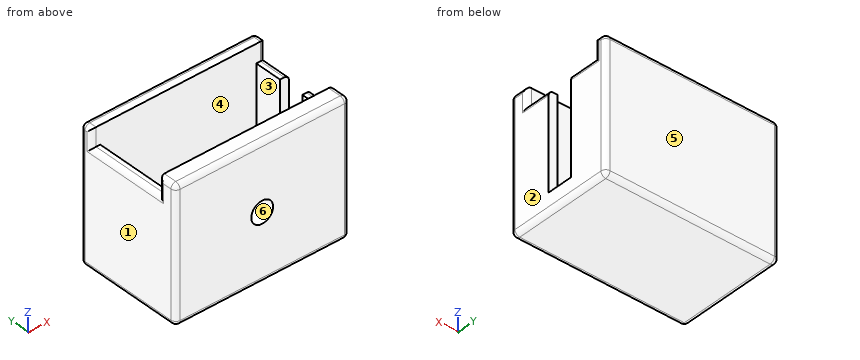
```python
from build123d import *

# Parameters (mm, degrees)
F0_W     = 46.0375
F0_H     = 28.575
F1_DEPTH = 4.7625
F3_DEPTH = 30.2895
F2_W     = 2.38125
F2_H     = 20.6375
F4_DEPTH = 25.4
F6_DEPTH = 2.38125
F8_D     = 5.7658
F8_DEPTH = 4.7625
F8_TIP   = 1.7322210786
F9_R     = 1.27


# Not quite as in the source:
# - a feature names something its author has since deleted; it is built from what else it names


with BuildPart() as f1:
    # F0 (on Top) → F1 (new body)
    with BuildSketch(Plane.XY):
        Rectangle(F0_W, F0_H)
    extrude(amount=F1_DEPTH)

    # F2 (on face) → F3 (join)
    with BuildSketch(Plane.XY.offset(4.7625)):
        Polygon((-23.01875, -9.525), (-23.01875, -14.2875), (23.01875, -14.2875), (23.01875, -9.525), (20.6375, -9.525), (-20.6375, -9.525), align=None)
        Polygon((-23.01875, 14.2875), (-23.01875, 11.1125), (-20.6375, 11.1125), (20.6375, 11.1125), (23.01875, 11.1125), (23.01875, 14.2875), align=None)
    extrude(amount=F3_DEPTH)

    # F2 (on face) → F4 (join)
    with BuildSketch(Plane.XY.offset(4.7625)):
        Polygon((-23.01875, -9.525), (-23.01875, -14.2875), (23.01875, -14.2875), (23.01875, -9.525), (20.6375, -9.525), (-20.6375, -9.525), align=None)
        with Locations((-21.828125, 0.79375)):
            Rectangle(F2_W, F2_H)
        with Locations((21.828125, 0.79375)):
            Rectangle(F2_W, F2_H)
        Polygon((-23.01875, 14.2875), (-23.01875, 11.1125), (-20.6375, 11.1125), (20.6375, 11.1125), (23.01875, 11.1125), (23.01875, 14.2875), align=None)
    extrude(amount=F4_DEPTH)

    # F5 (on face) → F6 (cut, through all)
    with BuildSketch(Plane.YZ.offset(23.01875)):
        Polygon((3.9749178039, 30.1625), (0.3463463753, 30.1625), (-2.8286536247, 30.1625), (-2.8286536247, 16.5712326925), (-2.8286536247, 11.8087326925), (-2.8286536247, 4.7625), (0.3463463753, 4.7625), (3.9749178039, 4.7625), (3.9749178039, 16.5712326925), align=None)
    extrude(amount=-F6_DEPTH, mode=Mode.SUBTRACT)

    # F8
    with Locations(Plane.XZ.offset(14.2875)):
        with Locations((0, 17.526)):
            Hole(F8_D / 2, depth=F8_DEPTH)
            with Locations((0, 0, -(F8_DEPTH + F8_TIP / 2))):  # 118° drill point
                Cone(0, F8_D / 2, F8_TIP, mode=Mode.SUBTRACT)

    # F9
    f9_edges = [f1.edges().sort_by_distance(p)[0] for p in [
        (23.01875, 14.2875, 17.526),
        (-23.01875, 14.2875, 17.526),
        (0, 14.2875, 35.052),
        (0, 14.2875, 0),
        (23.01875, 0, 0),
        (-23.01875, 0, 0),
        (23.01875, 12.7, 35.052),
        (-23.01875, 12.7, 35.052),
        (23.01875, -14.2875, 17.526),
        (0, -14.2875, 35.052),
        (-23.01875, -14.2875, 17.526),
        (0, -14.2875, 0),
        (23.01875, -11.90625, 35.052),
        (-23.01875, -11.90625, 35.052),
        (-23.01875, 0.79375, 30.1625),
        (23.01875, 7.543709, 30.1625),
        (23.01875, -6.176827, 30.1625),
        (23.01875, -9.525, 32.60725),
        (-23.01875, -9.525, 32.60725),
        (-23.01875, 11.1125, 32.60725),
        (23.01875, 11.1125, 32.60725),
    ]]
    fillet(f9_edges, radius=F9_R)


solid = f1.part
```
Part model, mm, in its own coordinate system. Face numbers are marked on the shaded views. A direction names the side the tool comes from. Coordinates: 2 decimals unless noted, no trailing zeros. Order: outer loops, then holes, each group sorted by start corner. A loop starts at its lowest first (then second) coordinate and runs counter-clockwise, first axis right, second up. Notation, with made-up numbers: (-2.5, 73) -> (39.5, 73) arc R20 ccw to (39.5, 81) -> close; hole circle Ø8 at (24.5, 24). An arc over 180 degrees is marked (long way). Put each result on its own line as item: value. Start each with the question number.
(1) Band-saw the part on C-C (y = 2.25). Give the cut face in (x, z), then the cut area to 3 significant figures.
(2) Pin check, flat tips, straight feed: pin 1 Ø0.6 at (x, y) = (21, -6.5) entering from +Z; pin 2 Ø1.2 at (x, z) = (22, 21) entering from -Y; pin 3 Ø1.2 at (x, z) = (22.5, 13) entering from +Y; pin 4 Ø1 at (x, y) = (7, 1.5) entering from +Z. Stop position of each tip, or through.
(3) Band-saw the part on D-D (z = 12.5). Give the cut face in (x, y) (1 decimal).
(4) Which spindle directions (+Z, -Z, +X, -X, +Y, -Y) get a long thin tool onto all of the face, cutting with end or side? Do the marked faces 4, 5 and 6. Say none if no direction does.
(5) Probe line 1 along X through (y, z) = (-3.5, 9); line 2 along Y through (x, z) = (18.5, 12) (1 decimal); line 3 along Z through (x, y) = (0, -12.85). List the from-to ranges inside material, lowest first. Write a range as [from, to].
(6) Band-saw the part on B-B (z = 17). Give the cut face in (x, y) (1 decimal), then the cut area to 3 significant figures.
(7) Band-saw the part on A-A (x = 0). Give the cut face in (y, z) (1 decimal).
(8) Mould opens along X. For the marked faces 1, 2 and 3 say: pulls with the +X half, pulls with the -X half, needs draft (parallel to the pull), parting line crosses it, or undercut.
Determined:
1. outline: (-23.02, 1.27) arc R1.27 ccw to (-21.75, 0) -> (21.75, 0) arc R1.27 ccw to (23.02, 1.27) -> (23.02, 4.76) -> (-20.64, 4.76) -> (-20.64, 30.16) -> (-21.75, 30.16) arc R1.27 ccw to (-23.02, 28.89) -> close
1. area: 279 mm²
2. pin 1: stops at z = 30.16
2. pin 2: stops at y = -14.29
2. pin 3: stops at y = 14.28
2. pin 4: stops at z = 4.76
3. outline: (-23, -13) arc R1.3 ccw to (-21.7, -14.3) -> (21.7, -14.3) arc R1.3 ccw to (23, -13) -> (23, -2.8) -> (20.6, -2.8) -> (20.6, -9.5) -> (-20.6, -9.5) -> (-20.6, 11.1) -> (20.6, 11.1) -> (20.6, 4) -> (23, 4) -> (23, 13) arc R1.3 ccw to (21.7, 14.3) -> (-21.7, 14.3) arc R1.3 ccw to (-23, 13) -> close
4. face 4: +Z
4. face 5: +Z, -Z, +X, -X, +Y
4. face 6: -Y
5. line 1: x = [-23.02, -20.64], [20.64, 23.02]
5. line 2: y = [-14.3, -9.5], [11.1, 14.3]
5. line 3: z = [0, 14.64], [20.41, 35.05]
6. outline: (-23, -13) arc R1.3 ccw to (-21.7, -14.3) -> (-2.8, -14.3) -> (-2.8, -9.5) -> (-20.6, -9.5) -> (-20.6, 11.1) -> (20.6, 11.1) -> (20.6, 4) -> (23, 4) -> (23, 13) arc R1.3 ccw to (21.7, 14.3) -> (-21.7, 14.3) arc R1.3 ccw to (-23, 13) -> close; (2.8, -14.3) -> (21.7, -14.3) arc R1.3 ccw to (23, -13) -> (23, -2.8) -> (20.6, -2.8) -> (20.6, -9.5) -> (2.8, -9.5) -> close
6. area: 419 mm²
7. outline: (-14.3, 1.3) arc R1.3 ccw to (-13, 0) -> (13, 0) arc R1.3 ccw to (14.3, 1.3) -> (14.3, 33.8) arc R1.3 ccw to (13, 35.1) -> (11.1, 35.1) -> (11.1, 4.8) -> (-9.5, 4.8) -> (-9.5, 14.6) -> (-14.3, 14.6) -> close; (-14.3, 20.4) -> (-9.5, 20.4) -> (-9.5, 35.1) -> (-13, 35.1) arc R1.3 ccw to (-14.3, 33.8) -> close
8. face 1: pulls with the -X half
8. face 2: pulls with the +X half
8. face 3: undercut
